Here's how the part is built. I have some questions about the finished solid (model axes, mm). Face numbers are marked on the shaded views. Coordinates: 2 decimals unless noted, no trailing zeros. Order: outer loops, then holes, each group sorted by start corner. A loop starts at its lowest first (then second) coordinate and runs counter-clockwise, first axis right, second up. Notation, with made-up numbers: (-9, 11) - (36, 11) arc R22 ccw to (36, 44) - close; hole circle Ø4 at (-26.5, 49). An arc over 180 degrees is marked (long way). Answer in a Markdown table with one row per item. Add a question column.
Item 1: Thinking about a two-plate mould opening in Y: for the marked faces 1, 2, 3 and 4, which applies, +Y half, -Y half, draft (parallel to the pull), parting line (faces both ways), or undercut?
Item 2: I want a section at B-B (x = 0). Please give me the cut outline in (y, z).
Item 3: I want a section at A-A (y = 0). Please give me the cut outline in (x, z).
Item 4: If I drill on line 1 along Y through (x, z) = (0, 1.15); line 2 along X through (y, z) = (4, 2.5); line 3 along Y through (x, z) = (5, 4.25), over which ranges is the centre line in solid material (lowest first)? Write a range as from..to.
Item 5: Will these pins go through, and if not, where does the flat tip stop? pin 1 Ø6.5 at (x, y) = (0, 17.5) entering from -Z; pin 2 Ø1 at (y, z) = (11.5, 4) entering from +X; pin 3 Ø18.5 at (x, y) = (0, 0) entering from +Z; pin 4 Ø3 at (y, z) = (11.5, 1.5) entering from -X.
Item 6: I want a section at D-D (y = -8.75). Please give me the cut outline in (x, z).
Item 7: I want a section at C-C (x = -7). Please give me the cut outline in (y, z).
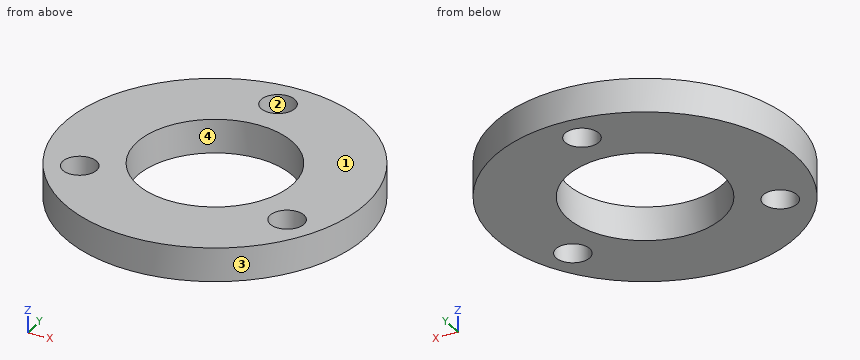
Autodesk Inventor part; units mm, degrees
ref_plane "YZ Plane" through (0, 0, 0) normal (1, 0, 0) x (0, 1, 0)
ref_plane "XZ Plane" through (0, 0, 0) normal (0, 1, 0) x (-1, 0, 0)
ref_plane "XY Plane" through (0, 0, 0) normal (0, 0, 1) x (1, 0, 0)
sketch "Sketch1" plane through (0, 0, 0) normal (0, 0, 1) x (1, 0, 0)
  circle A0 centre (0, 0) radius 11.5
  circle A1 centre (0, 0) radius 22.25
  circle A2 centre (0, 17.5) radius 2.5
  circle A3 centre (-15.1554, -8.75) radius 2.5
  circle A4 centre (15.1554, -8.75) radius 2.5
  dimension "d0" = 23
  dimension "d1" = 44.5
  dimension "d2" = 5
  dimension "d3" = 17.5
  dimension "d6" = 360
extrude "Extrusion1" add sketch "Sketch1" along normal blind 5
properties part number "TA06" material "ABS Plastic"
Values follow:
| question | item | result |
|---|---|---|
| 1 | face 1 | draft |
| 1 | face 2 | undercut |
| 1 | face 3 | parting line |
| 1 | face 4 | undercut |
| 2 | outline | (-22.25, 0) - (-11.5, 0) - (-11.5, 5) - (-22.25, 5) - close; (11.5, 0) - (15, 0) - (15, 5) - (11.5, 5) - close; (20, 0) - (22.25, 0) - (22.25, 5) - (20, 5) - close |
| 3 | outline | (-22.25, 0) - (-11.5, 0) - (-11.5, 5) - (-22.25, 5) - close; (11.5, 0) - (22.25, 0) - (22.25, 5) - (11.5, 5) - close |
| 4 | line 1 | y = -22.25..-11.5, 11.5..15, 20..22.25 |
| 4 | line 2 | x = -21.89..-10.78, 10.78..21.89 |
| 4 | line 3 | y = -21.68..-10.36, 10.36..21.68 |
| 5 | pin 1 | stops at z = 0 |
| 5 | pin 2 | stops at x = 19.34 |
| 5 | pin 3 | passes through |
| 5 | pin 4 | stops at x = -19.88 |
| 6 | outline | (-20.46, 0) - (-17.66, 0) - (-17.66, 5) - (-20.46, 5) - close; (-12.66, 0) - (-7.46, 0) - (-7.46, 5) - (-12.66, 5) - close; (7.46, 0) - (12.66, 0) - (12.66, 5) - (7.46, 5) - close; (17.66, 0) - (20.46, 0) - (20.46, 5) - (17.66, 5) - close |
| 7 | outline | (-21.12, 0) - (-9.12, 0) - (-9.12, 5) - (-21.12, 5) - close; (9.12, 0) - (21.12, 0) - (21.12, 5) - (9.12, 5) - close |
